from build123d import *

# Parameters (mm, degrees)
BOSS_EXTRUDE1_DEPTH   = 7
SKETCH2_R             = 5
BOSS_EXTRUDE2_DEPTH   = 40
M6_TAPPED_HOLE1_D     = 5
M6_TAPPED_HOLE1_DEPTH = 15
M6_TAPPED_HOLE1_TIP   = 1.502151548


with BuildPart() as part:
    # Sketch1 → Boss-Extrude1 (new body)
    with BuildSketch(Plane.XY):
        with BuildLine():
            Line((-9, 50), (-9, 0))
            ThreePointArc((-9, 0), (0, -9), (9, 0))
            Line((9, 0), (9, 50))
            ThreePointArc((9, 50), (0, 59), (-9, 50))
        make_face()
    extrude(amount=BOSS_EXTRUDE1_DEPTH)

    # Sketch2 → Boss-Extrude2 (add)
    with BuildSketch(Plane.XY.offset(7)):
        with Locations(Location((0, 0, 0), (0, 0, 180))):  # turned: the seam where the file's is
            Circle(SKETCH2_R)
    extrude(amount=BOSS_EXTRUDE2_DEPTH)

    # M6 Tapped Hole1
    with Locations(Plane(origin=(0, 0, 0), x_dir=(-1, 0, 0), z_dir=(0, 0, -1))):
        with Locations((0, 50)):
            Hole(M6_TAPPED_HOLE1_D / 2, depth=M6_TAPPED_HOLE1_DEPTH)
            with Locations((0, 0, -(M6_TAPPED_HOLE1_DEPTH + M6_TAPPED_HOLE1_TIP / 2))):  # 118° drill point
                Cone(0, M6_TAPPED_HOLE1_D / 2, M6_TAPPED_HOLE1_TIP, mode=Mode.SUBTRACT)


solid = part.part
Read the model definition and answer for the solid it produces. Units are mm, in the model's axes. A direction names the side the tool comes from. Coordinates: 2 decimals unless noted, no trailing zeros. Loops run counter-clockwise (first coordinate to the right, second up) from the corner with the lowest first, then second, coordinate; pieces in that order, holes last. Notation, with made-up numbers: (50.5, 66.25) - (77.5, 66.25) arc R20 ccw to (77.5, 92.25) - close; hole circle Ø6 at (-22, 52.5). An arc over 180 degrees is marked (long way). Answer in a Markdown table with one row per item.
Q1. Find section D-D on x = -3.25. Write down the section's boundary in (y, z), plus the area to 3 significant figures.
Here are the results:
| item | result |
|---|---|
| outline | (-8.39, 0) - (58.39, 0) - (58.39, 7) - (3.8, 7) - (3.8, 47) - (-3.8, 47) - (-3.8, 7) - (-8.39, 7) - close |
| area | 771 mm^2 |
Q2. Straight lines are drawn through the part: line 1 along Y through (x, z) = (0, 3); line 2 along Z through (x, y) = (-4.75, 55); line 3 along Y through (x, z) = (-7.75, 3.5). For each, find the intervals that lie inside material, in ascending order. Write a range as [from, to].
Here are the results:
| item | result |
|---|---|
| line 1 | y = [-9, 47.5], [52.5, 59] |
| line 2 | z = [0, 7] |
| line 3 | y = [-4.58, 54.58] |
Q3. For faces 1 (the flat face through (0, 0, 47)), 2 (the cylindrical face through (5, 0, 27)), determine the directions among +Z, -Z, +X, -X, +Y, -Y from which every point of the face is accessible in a straight line to the end or side of a thin tool.
Here are the results:
| item | result |
|---|---|
| face 1 | +Z, +X, -X, +Y, -Y |
| face 2 | +Z |
Q4. The mould has two halves that part along Y. Classify faces 3 (the flat face through (0, 25, 0)), 4 (the cylindrical face through (-0.54, 47.56, 3.55)), 5 (the cylindrical face through (0, -9, 3)): pulls with the +Y half, pulls with the -Y half, needs draft (parallel to the pull), parting line crosses it, or undercut.
Here are the results:
| item | result |
|---|---|
| face 3 | needs draft |
| face 4 | undercut |
| face 5 | pulls with the -Y half |
Q5. Find section C-C on y = 31. Write down the section's boundary in (x, z).
Here are the results:
| item | result |
|---|---|
| outline | (-9, 0) - (9, 0) - (9, 7) - (-9, 7) - close |
Q6. Find section B-B on z = 4.5. Write down the section's boundary in (x, y), plus the area to 3 significant figures.
Here are the results:
| item | result |
|---|---|
| outline | (-9, 0) arc R9 ccw to (9, 0) - (9, 50) arc R9 ccw to (-9, 50) - close; hole circle Ø5 at (0, 50) |
| area | 1,130 mm^2 |
Q7. Given P1, Ø4, axis at x = 3.5, z = 24, coming from the +Y side; P2, Ø1.5, axis at x = 6.5, z = 28.5, coming from the -Y side; P3, Ø2, axis at x = 6, y = 28.5, coming from the +Z side; P4, Ø4, axis at x = 5.5, z = 39, coming from the +Y side, each flat-ended and moving along its own axis, determine where each tip first touches the part or whether it passes through.
Here are the results:
| item | result |
|---|---|
| P1 | stops at y = 4.77 |
| P2 | passes through |
| P3 | stops at z = 7 |
| P4 | stops at y = 3.57 |
Q8. Find section A-A on x = 0.5. Write down the section's boundary in (y, z), plus the area to 3 significant figures.
Here are the results:
| item | result |
|---|---|
| outline | (-8.99, 0) - (47.55, 0) - (47.55, 7) - (4.97, 7) - (4.97, 47) - (-4.97, 47) - (-4.97, 7) - (-8.99, 7) - close; (52.45, 0) - (58.99, 0) - (58.99, 7) - (52.45, 7) - close |
| area | 840 mm^2 |
